Input: part model. Units: mm. Frame: model coordinates. Round coordinates to 2 decimals unless told otherwise and drop trailing zeros. Loops run counter-clockwise (first coordinate to the right, second up) from the corner with the lowest first, then second, coordinate; pieces in that order, holes last.
(1) Cut plane C-C, the plane x = -10.5. Output: boundary loops of the cut face in (y, z) (3 decimals).
(2) Cut plane B-B, the plane z = 6.5. Output: boundary loops of the cut face in (x, y), and give its area (3 significant figures).
(3) Line query: line 1 (Z direction, x = -3, y = 0.35). Output: solid intervals per line, ascending.
(4) First-contact query: pin 1 Ø2.5 at (x, z) = (-7, -5) entering from +Y; pin 2 Ø1 at (x, z) = (-6.5, 5.5) entering from -Y. Flat tips, straight axial feed; report the tip coordinate or a pass-through.
(5) Draft query along Y for faces 1 (the face through (-8, 0, 8)), 2 (the face through (-7, 0.5, -5)), 3 (the face through (-7, 0.3, 5)), 4 (the face through (-8, 0.8, -8)). Return one class per face: released by +Y, released by -Y, zero draft, split by the parting line, or undercut.
(6) Cut plane A-A, the plane x = -3.25. Output: boundary loops of the cut face in (y, z) (3 decimals), and give its area (3 significant figures).
(7) Cut plane D-D, the plane z = -5. Output: boundary loops of the cut face in (x, y), and give its area (3 significant figures).
from build123d import *

# Parameters (mm, degrees)
BOSS_EXTRUDE1_DEPTH = 0.8
CUT_EXTRUDE1_START  = -5.3
CUT_EXTRUDE1_DEPTH  = 21.7
SKETCH3_W           = 15
SKETCH3_H           = 20.9
CUT_EXTRUDE2_DEPTH  = 1.8


with BuildPart() as part:
    # Sketch1 → Boss-Extrude1 (new body)
    with BuildSketch(Plane(origin=(0, 0, 0), x_dir=(1, 0, 0), z_dir=(0, 1, 0))):
        Polygon((13.478240741, 10.45), (-13.478240741, 10.45), (-13.478240741, -10.45), (13.478240741, -10.45), (13.478240741, -0.35), (-8.221759259, -0.35), (-8.221759259, 0.35), (13.478240741, 0.35), align=None)
    extrude(amount=BOSS_EXTRUDE1_DEPTH)

    # Sketch2 → Cut-Extrude1 (cut)
    with BuildSketch(Plane(origin=(13.478240741, 0, 0), x_dir=(0, 0, -1), z_dir=(1, 0, 0)).offset(CUT_EXTRUDE1_START)):
        Polygon((-7.025, 0.5), (-3.775, 0.5), (-4.525, 0.8), (-6.275, 0.8), align=None)
        Polygon((-7.025, 0.3), (-6.275, 0), (-4.525, 0), (-3.775, 0.3), align=None)
        Polygon((7.025, 0.3), (3.775, 0.3), (4.525, 0), (6.275, 0), align=None)
        Polygon((7.025, 0.5), (6.275, 0.8), (4.525, 0.8), (3.775, 0.5), align=None)
    extrude(amount=-CUT_EXTRUDE1_DEPTH, mode=Mode.SUBTRACT)

    # Sketch3 → Cut-Extrude2 (cut, through all)
    with BuildSketch(Plane(origin=(0, 0.8, 0), x_dir=(1, 0, 0), z_dir=(0, 1, 0))):
        with Locations((5.978240741, 0)):
            Rectangle(SKETCH3_W, SKETCH3_H)
    extrude(amount=-CUT_EXTRUDE2_DEPTH, mode=Mode.SUBTRACT)


solid = part.part
Reported:
1. outline: (0, -10.45) - (0.8, -10.45) - (0.8, -6.275) - (0.5, -7.025) - (0.5, -3.775) - (0.8, -4.525) - (0.8, 4.525) - (0.5, 3.775) - (0.5, 7.025) - (0.8, 6.275) - (0.8, 10.45) - (0, 10.45) - (0, 6.275) - (0.3, 7.025) - (0.3, 3.775) - (0, 4.525) - (0, -4.525) - (0.3, -3.775) - (0.3, -7.025) - (0, -6.275) - close
2. outline: (-13.48, 0) - (-1.52, 0) - (-1.52, 0.09) - (-13.48, 0.09) - close; (-13.48, 0.3) - (-1.52, 0.3) - (-1.52, 0.5) - (-13.48, 0.5) - close; (-13.48, 0.71) - (-1.52, 0.71) - (-1.52, 0.8) - (-13.48, 0.8) - close
2. area: 4.54 mm2
3. line 1: z = -10.45 to -0.35, 0.35 to 10.45
4. pin 1: stops at y = 0.8
4. pin 2: stops at y = 0.3
5. face 1: released by -Y
5. face 2: undercut
5. face 3: undercut
5. face 4: released by +Y
6. outline: (0, -10.45) - (0.8, -10.45) - (0.8, -6.275) - (0.5, -7.025) - (0.5, -3.775) - (0.8, -4.525) - (0.8, -0.35) - (0, -0.35) - (0, -4.525) - (0.3, -3.775) - (0.3, -7.025) - (0, -6.275) - close; (0, 0.35) - (0.8, 0.35) - (0.8, 4.525) - (0.5, 3.775) - (0.5, 7.025) - (0.8, 6.275) - (0.8, 10.45) - (0, 10.45) - (0, 6.275) - (0.3, 7.025) - (0.3, 3.775) - (0, 4.525) - close
6. area: 13.2 mm2
7. outline: (-13.48, 0.3) - (-1.52, 0.3) - (-1.52, 0.5) - (-13.48, 0.5) - close
7. area: 2.39 mm2
